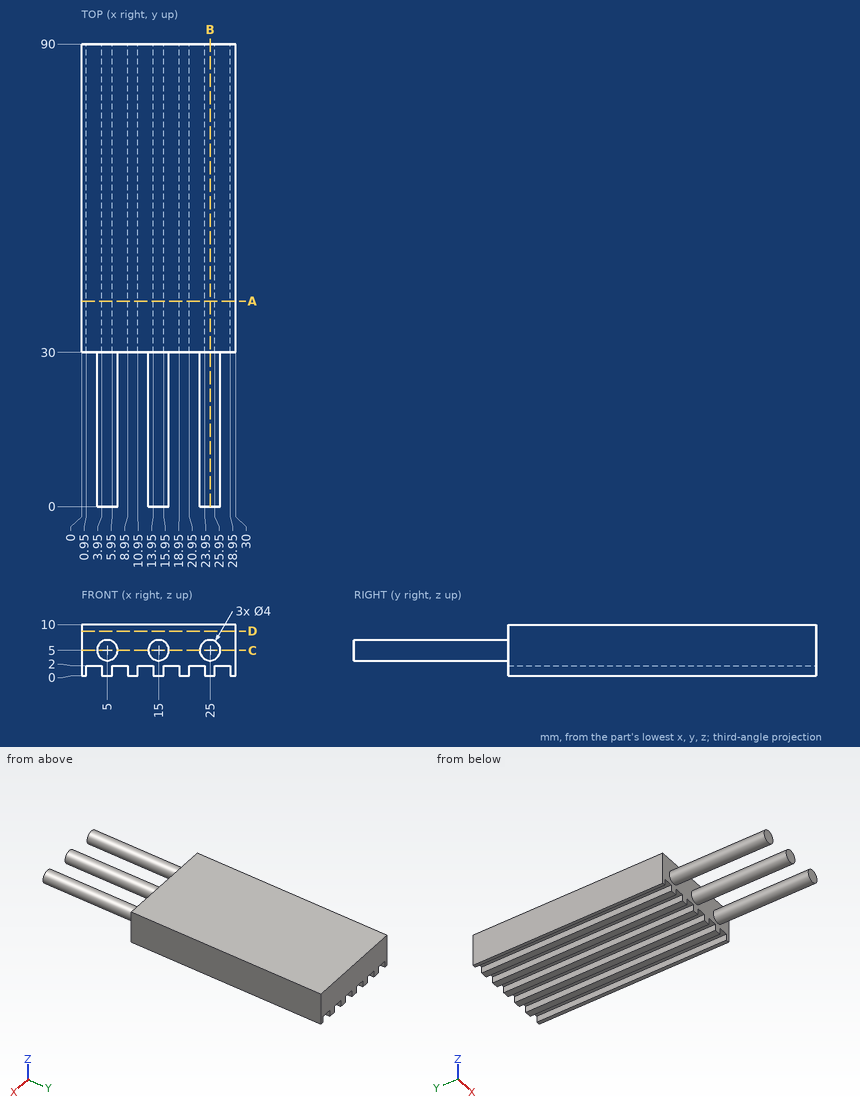
Answer from the drawing. Dimensions are ordinates in mm from the lowest x, y and z of the part. Give positions to 0.01 mm unless a question says otherwise; leave off trailing zeros. Order: outer loops, then holes, each group sorted by start corner. A loop starts at its lowest first (then second) coordinate and runs counter-clockwise, first axis right, second up. Notation, with made-up numbers: (-32.5, 58) - (6.5, 58) arc R10 ccw to (6.5, 68) - close; hole circle Ø9 at (49, 23.25). An arc over 180 degrees is marked (long way). One line per item, written item: value. Start each with the question number.
1. Section A-A, the plane y = 40 is taken. Write down the section's boundary in (x, z).
2. Section D-D, the plane z = 8.75 is taken. Write down the section's boundary in (x, y).
3. Each of these flat-tipped pins is pushed along its axis until it touches: pin 1 Ø2 at (y, z) = (35.5, 3) entering from -X; pin 2 Ø1.5 at (x, y) = (28, 50) entering from -Z; pin 3 Ø1.5 at (x, y) = (3.5, 17) entering from -Z; pin 4 Ø10 at (x, y) = (6, 16.5) entering from -Z. Where does it stop, or does it pass through?
4. Section B-B, the plane x = 25 is taken. Write down the section's boundary in (y, z).
5. Consider line 1 (X direction, y = 22, z = 6.5) (1 decimal); line 2 (Y direction, x = 7.25, z = 4.5); line 3 (Z direction, x = 27, y = 48.5). Determine where each line is inside the solid, lowest interval first.
6. Section C-C, the plane z = 5 is taken. Write down the section's boundary in (x, y), then the cut area to 3 significant figures.
Filled sheet:
1. outline: (0, 0) - (0.95, 0) - (0.95, 2) - (3.95, 2) - (3.95, 0) - (5.95, 0) - (5.95, 2) - (8.95, 2) - (8.95, 0) - (10.95, 0) - (10.95, 2) - (13.95, 2) - (13.95, 0) - (15.95, 0) - (15.95, 2) - (18.95, 2) - (18.95, 0) - (20.95, 0) - (20.95, 2) - (23.95, 2) - (23.95, 0) - (25.95, 0) - (25.95, 2) - (28.95, 2) - (28.95, 0) - (30, 0) - (30, 10) - (0, 10) - close
2. outline: (0, 30) - (30, 30) - (30, 90) - (0, 90) - close
3. pin 1: x = 0
3. pin 2: z = 2
3. pin 3: z = 3.15
3. pin 4: z = 3
4. outline: (0, 3) - (30, 3) - (30, 0) - (90, 0) - (90, 10) - (30, 10) - (30, 7) - (0, 7) - close
5. line 1: 3.7 to 6.3, 13.7 to 16.3, 23.7 to 26.3
5. line 2: 30 to 90
5. line 3: 2 to 10
6. outline: (0, 30) - (3, 30) - (3, 0) - (7, 0) - (7, 30) - (13, 30) - (13, 0) - (17, 0) - (17, 30) - (23, 30) - (23, 0) - (27, 0) - (27, 30) - (30, 30) - (30, 90) - (0, 90) - close
6. area: 2,160 mm²
